from build123d import *

# Parameters (mm, degrees)
F0_R     = 3
F0_R_2   = 11
F0_W     = 40
F0_H     = 9
F1_DEPTH = 12
F2_DEPTH = 4
F3_R     = 5
F4_R     = 1


with BuildPart() as f1:
    # F0 (on Top) → F1 (new body)
    with BuildSketch(Plane.XY):
        Polygon((40, 0), (0, 0), (0, -13), (0, -26), (40, -26), (40, -13), align=None)
        with Locations((5, -19.5)):
            Circle(F0_R, mode=Mode.SUBTRACT)
        with Locations((35, -19.5)):
            Circle(F0_R, mode=Mode.SUBTRACT)
        with Locations((5, -6.5)):
            Circle(F0_R, mode=Mode.SUBTRACT)
        with Locations((20, -13)):
            Circle(F0_R_2, mode=Mode.SUBTRACT)
        with Locations((35, -6.5)):
            Circle(F0_R, mode=Mode.SUBTRACT)
        with Locations((20, -13)):
            Circle(F0_R_2)
        with Locations((20, -30.5)):
            Rectangle(F0_W, F0_H)
        with Locations((5, -30.5)):
            Circle(F0_R, mode=Mode.SUBTRACT)
        with Locations((16, -30.5)):
            Circle(F0_R, mode=Mode.SUBTRACT)
        with Locations((24, -30.5)):
            Circle(F0_R, mode=Mode.SUBTRACT)
        with Locations((35, -30.5)):
            Circle(F0_R, mode=Mode.SUBTRACT)
    extrude(amount=F1_DEPTH)

    # F0 (on Top) → F2 (cut)
    with BuildSketch(Plane.XY):
        with Locations((20, -13)):
            Circle(F0_R_2)
    extrude(amount=F2_DEPTH, mode=Mode.SUBTRACT)

    # F3
    f3_edges = [f1.edges().sort_by_distance(p)[0] for p in [
        (40, -35, 6),
        (0, -35, 6),
        (0, 0, 6),
        (40, 0, 6),
    ]]
    fillet(f3_edges, radius=F3_R)

    # F4
    f4_edges = [f1.edges().sort_by_distance(p)[0] for p in [
        (9, -13, 4),
        (9, -13, 0),
    ]]
    fillet(f4_edges, radius=F4_R)


solid = f1.part
Source: CAD feature listing. Evaluate the final solid. Frame: model axes, mm. A direction names the side the tool comes from. Round coordinates to 2 decimals unless told otherwise and drop trailing zeros. Loops run counter-clockwise (first coordinate to the right, second up) from the corner with the lowest first, then second, coordinate; pieces in that order, holes last. Notation, with made-up numbers: M 0,16.25 L 43,16.25 A24 cw 43,54.25 Z; hole C 55,56 d10. An arc over 180 degrees is marked long. Return JSON: item names as keys, results as strings. Group by question number.
1. Section query A-A on z = 6.75. State how many separate pieces and enclosed holes the cut face has, and give its area (3 significant figures).
2. Section query B-B on x = 20. Output: boundary loops of the cut face in (y, z), and give its area (3 significant figures).
3. Mould query, pull axis Y, two halves, no side actions, for faces 1 (the face through (21, -30.4, 5.9)), 2 (the face through (20, -35, 6)), 3 (the face through (38, -1, 6)), 4 (the face through (4.35, -33.43, 5.92)). Classes: released by +Y, released by -Y, zero draft, split by the parting line, or undercut.
4. Reachability of faces 5 (the face through (2, -1, 6)), 6 (the face through (30.161, -17.213, 1.986)) from +Z, -Z, +X, -X, +Y, -Y: full face, straight path, thin tool, end or side. Return the list, or none.
5. Material intervals for line 1 along Y through (x, z) = (35, 3.5); line 2 along X through (y, z) = (-17, 10); line 3 along X through (y, z) = (-8.5, 2.5), sorted ascending. Write a range as from..to.
6. Section query D-D on x = 34. Output: boundary loops of the cut face in (y, z).
7. Pin query (flat end, axial travel): pin 1 (5.5 mm diameter, centred on x = 16, y = -30.5, fed in from -Z); pin 2 (8 mm diameter, centred on x = 35, y = -30.5, fed in from +Z); pin 3 (10 mm diameter, centred on x = 18, y = -9.5, fed in from -Z). Return the tip coordinate at first contact, or that it passes through.
Checks:
{
 "1": {"separate pieces": "1", "enclosed holes": "8", "area": "1,150 mm²"},
 "2": {"outline": "M -35,0 L -25,0 A1 ccw -24,1 L -24,3 A1 cw -23,4 L -3,4 A1 cw -2,3 L -2,1 A1 ccw -1,0 L 0,0 L 0,12 L -35,12 Z", "area": "332 mm²"},
 "3": {"face 1": "undercut", "face 2": "released by -Y", "face 3": "released by +Y", "face 4": "undercut"},
 "4": {"face 5": "+Z, -Z, -X, +Y", "face 6": "-Z"},
 "5": {"line 1": "y = -35..-33.5, -27.5..-22.5, -16.5..-9.5, -3.5..0", "line 2": "x = 0..3.34, 6.66..33.34, 36.66..40", "line 3": "x = 0..2.76, 7.24..9.96, 30.04..32.76, 37.24..40"},
 "6": {"outline": "M -35,0 L -33.33,0 L -33.33,12 L -35,12 Z; M -27.67,0 L -22.33,0 L -22.33,12 L -27.67,12 Z; M -16.67,0 L -9.33,0 L -9.33,12 L -16.67,12 Z; M -3.67,0 L 0,0 L 0,12 L -3.67,12 Z"},
 "7": {"pin 1": "passes through", "pin 2": "stops at z = 12", "pin 3": "stops at z = 4"}
}
